```python
from build123d import *

# Parameters (mm, degrees)
SKETCH1_W               = 34.67
SKETCH1_H               = 34.29
BOSS_EXTRUDE1_DEPTH     = 1
SKETCH3_W               = 3.5
SKETCH3_H               = 34.29
BOSS_EXTRUDE2_DEPTH     = 5
CUT_EXTRUDE1_DEPTH      = 26.108828129
CUT_EXTRUDE1_DEPTH_BACK = 26.108828129
SKETCH5_W               = 1.5
SKETCH5_H               = 30
SKETCH6_W               = 3
SKETCH6_H               = 4.2
SKETCH6_W_2             = 8.11
SKETCH6_H_2             = 7
BOSS_EXTRUDE3_DEPTH     = 2.1
FILLET1_R               = 1.5
CUT_EXTRUDE2_DEPTH      = 25.577698224
CUT_EXTRUDE2_DEPTH_BACK = 25.577698224
SKETCH7_R               = 0.8
CHAMFER1_SIZE           = 0.3


with BuildPart() as part:
    # Sketch1 → Boss-Extrude1 (new body)
    with BuildSketch(Plane.YZ):
        Rectangle(SKETCH1_W, SKETCH1_H)
    extrude(amount=BOSS_EXTRUDE1_DEPTH)

    # Sketch3 → Boss-Extrude2 (add)
    with BuildSketch(Plane.YZ.offset(1)):
        with Locations((-15.585, 0)):
            Rectangle(SKETCH3_W, SKETCH3_H)
        with Locations((15.585, 0)):
            Rectangle(SKETCH3_W, SKETCH3_H)
    extrude(amount=BOSS_EXTRUDE2_DEPTH)

    # Sketch5 → Cut-Extrude1 (cut, two sides: drawn at the far end of the back side and taken through both)
    with BuildSketch(Plane.YZ.offset(6).offset(-CUT_EXTRUDE1_DEPTH_BACK)):
        with Locations((-15.585, 0)):
            Rectangle(SKETCH5_W, SKETCH5_H)
        with Locations((15.585, 0)):
            Rectangle(SKETCH5_W, SKETCH5_H)
    extrude(amount=CUT_EXTRUDE1_DEPTH + CUT_EXTRUDE1_DEPTH_BACK, mode=Mode.SUBTRACT)

    # Sketch6 → Boss-Extrude3 (add)
    with BuildSketch(Plane.YZ.offset(1)):
        with Locations((-12.335, 5.745)):
            Rectangle(SKETCH6_W, SKETCH6_H)
        with Locations((-9.78, -13.645)):
            Rectangle(SKETCH6_W_2, SKETCH6_H_2)
        with Locations((9.78, -13.645)):
            Rectangle(SKETCH6_W_2, SKETCH6_H_2)
        with Locations((12.335, 5.745)):
            Rectangle(SKETCH6_W, SKETCH6_H)
    extrude(amount=BOSS_EXTRUDE3_DEPTH)

    # Fillet1
    fillet1_edges = [part.edges().sort_by_distance(p)[0] for p in [
        (2.05, 5.725, -10.145),
        (2.05, -5.725, -10.145),
        (2.05, -10.835, 3.645),
        (2.05, -10.835, 7.845),
        (2.05, 10.835, 7.845),
        (2.05, 10.835, 3.645),
    ]]
    fillet(fillet1_edges, radius=FILLET1_R)

    # Sketch7 → Cut-Extrude2 (cut, two sides: drawn at the far end of the back side and taken through both)
    with BuildSketch(Plane.YZ.offset(3.1).offset(-CUT_EXTRUDE2_DEPTH_BACK)):
        with Locations(Location((-9.525, -13.335, 0), (0, 0, 270))):
            Circle(SKETCH7_R)
        with Locations(Location((9.525, -13.335, 0), (0, 0, 270))):
            Circle(SKETCH7_R)
    extrude(amount=CUT_EXTRUDE2_DEPTH + CUT_EXTRUDE2_DEPTH_BACK, mode=Mode.SUBTRACT)

    # Chamfer1
    chamfer1_edges = [part.edges().sort_by_distance(p)[0] for p in [
        (0, -9.525, -12.535),
        (0, 9.525, -12.535),
        (0, 0, -17.145),
        (0, -17.335, 0),
        (0, -14.835, 0),
        (0, -15.585, -15),
        (0, -16.335, 0),
        (0, -15.585, 15),
        (0, 0, 17.145),
        (0, 16.335, 0),
        (0, 15.585, -15),
        (0, 14.835, 0),
        (0, 17.335, 0),
        (0, 15.585, 15),
    ]]
    chamfer(chamfer1_edges, length=CHAMFER1_SIZE)


solid = part.part
```
Design review of the part built by this model. Coordinates are the model's own, in mm. A direction names the side the tool comes from. Round coordinates to 2 decimals unless told otherwise and drop trailing zeros. Write each loop counter-clockwise with the first axis right and the second up, starting at its lowest first coordinate (ties: lowest second). Pieces come first, ordered by that corner, then holes. Notation, with made-up numbers: (41.5, 60.5) -> (59.5, 60.5) arc R5 ccw to (59.5, 68.5) -> close; hole circle Ø2 at (11, 56.5). An arc over 180 degrees is marked (long way). Answer in a Markdown table with one row per item.
Q1. Take a section at D-D, the plane x = 1.5. Count the separate pieces of the cut face and the enclosed holes in it, then the cut area to 3 significant figures.
The answers:
| item | result |
|---|---|
| separate pieces | 2 |
| enclosed holes | 4 |
| area | 282 mm² |
Q2. Clearance check with flat-ended pins moving along their axes: pin 1 Ø1.7 at (x, y) = (2, -9.5) entering from +Z (3 decimals); pin 2 Ø2 at (y, z) = (9.525, -13.335) entering from -X; pin 3 Ø6 at (y, z) = (6, 12) entering from +X. State where each tip first meets the part, or that it passes through.
The answers:
| item | result |
|---|---|
| pin 1 | z = -10.145 |
| pin 2 | x = 0.1 |
| pin 3 | x = 1 |
Q3. Take a section at A-A, the plane x = 3.75. State the section outline as (y, z) points (3 decimals), then the cut area to 3 significant figures.
The answers:
| item | result |
|---|---|
| outline | (-17.335, -17.145) -> (-13.835, -17.145) -> (-13.835, 17.145) -> (-17.335, 17.145) -> close; (13.835, -17.145) -> (17.335, -17.145) -> (17.335, 17.145) -> (13.835, 17.145) -> close; hole (-16.335, -15) -> (-14.835, -15) -> (-14.835, 15) -> (-16.335, 15) -> close; hole (14.835, -15) -> (16.335, -15) -> (16.335, 15) -> (14.835, 15) -> close |
| area | 150 mm² |
Q4. Draft analysis for pull direction Z (two halves, no side actions). For faces 1 (the face through (3, 17.335, 0)), 2 (the face through (2.06, 11.29, 7.42)), 3 (the face through (3, 13.835, 0)), state which applies: +Z half, -Z half, draft (parallel to the pull), parting line (faces both ways), or undercut.
The answers:
| item | result |
|---|---|
| face 1 | draft |
| face 2 | +Z half |
| face 3 | undercut |
Q5. For faces 4 (the face through (2, 10, -10.145)), 5 (the face through (3, -14.835, 0)), 6 (the face through (2, -13, 7.845)), 7 (the face through (3.1, -9.8, -14.4)), list the 3-axis set-ups (+Z, -Z, +X, -X, +Y, -Y) from which the entire face can be reached by the end or side of a thin tool; tool diameter is ignored.
The answers:
| item | result |
|---|---|
| face 4 | +X |
| face 5 | +X, -X |
| face 6 | +Z, +X |
| face 7 | +Z, -Z, +X |
Q6. To check wall thickness, follow L1, parallel to Y at x = 5.5, z = 3.5 (3 decimals); L2, parallel to Y at x = 1.75, z = 5.5 (3 decimals); L3, parallel to Y at x = 0.5, z = -3.5 (3 decimals). State the ranges of each line that lie inside material, in increasing order. Write a range as [from, to].
The answers:
| item | result |
|---|---|
| L1 | [-17.335, -16.335], [-14.835, -13.835], [13.835, 14.835], [16.335, 17.335] |
| L2 | [-17.335, -16.335], [-14.835, -10.835], [10.835, 14.835], [16.335, 17.335] |
| L3 | [-17.335, -16.335], [-14.835, 14.835], [16.335, 17.335] |
Q7. Take a section at B-B, the plane z = 9.5. State the section outline as (x, y) points (3 decimals), then the cut area to 3 significant figures.
The answers:
| item | result |
|---|---|
| outline | (0, -17.035) -> (0.3, -17.335) -> (6, -17.335) -> (6, -16.335) -> (0.3, -16.335) -> (0, -16.635) -> close; (0, -14.535) -> (0.3, -14.835) -> (6, -14.835) -> (6, -13.835) -> (1, -13.835) -> (1, 13.835) -> (6, 13.835) -> (6, 14.835) -> (0.3, 14.835) -> (0, 14.535) -> close; (0, 16.635) -> (0.3, 16.335) -> (6, 16.335) -> (6, 17.335) -> (0.3, 17.335) -> (0, 17.035) -> close |
| area | 51.4 mm² |
Q8. Take a section at C-C, the plane y = 1. State the section outline as (x, z) points (3 decimals), then the cut area to 3 significant figures.
The answers:
| item | result |
|---|---|
| outline | (0, -16.845) -> (0.3, -17.145) -> (1, -17.145) -> (1, 17.145) -> (0.3, 17.145) -> (0, 16.845) -> close |
| area | 34.2 mm² |
